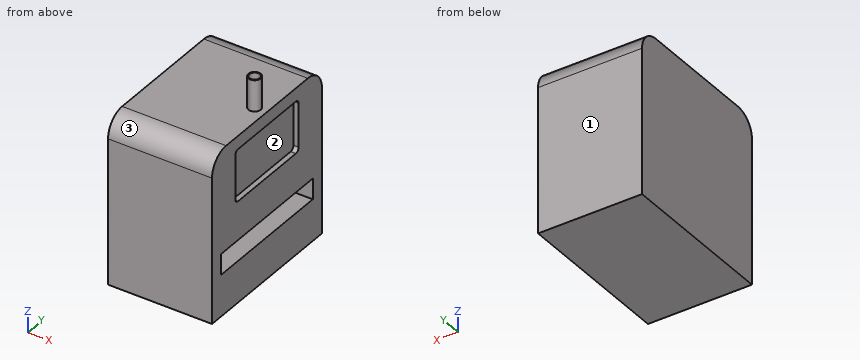
```python
from build123d import *

# Parameters (mm, degrees)
F0_W      = 780
F0_H      = 800
F1_DEPTH  = 500
F2_R      = 100
F3_R      = 30
F4_DEPTH  = 150
F5_R      = 25
F6_DEPTH  = 200
F7_W      = 450
F7_H      = 250
F8_DEPTH  = 25
F9_R      = 20
F11_DEPTH = 150


with BuildPart() as f1:
    # F0 (on Right) → F1 (new body)
    with BuildSketch(Plane.YZ):
        Rectangle(F0_W, F0_H)
    extrude(amount=-F1_DEPTH)

    # F2
    f2_edges = [f1.edges().sort_by_distance(p)[0] for p in [
        (-250, -390, 400),
        (-250, 390, 400),
    ]]
    fillet(f2_edges, radius=F2_R)

    # F3 (on face) → F4 (join)
    with BuildSketch(Plane.XY.offset(400)):
        with Locations((-59.408359, 0)):
            Circle(F3_R)
    extrude(amount=F4_DEPTH)

    # F5 (on face) → F6 (cut)
    with BuildSketch(Plane.XY.offset(550)):
        with Locations((-59.408359, 0)):
            Circle(F5_R)
    extrude(amount=-F6_DEPTH, mode=Mode.SUBTRACT)

    # F7 (on face) → F8 (cut)
    with BuildSketch(Plane.YZ):
        with Locations((0, 211.28722)):
            Rectangle(F7_W, F7_H)
    extrude(amount=-F8_DEPTH, mode=Mode.SUBTRACT)

    # F9
    f9_edges = [f1.edges().sort_by_distance(p)[0] for p in [
        (-12.5, -225, 336.28722),
        (-12.5, 225, 336.28722),
        (-12.5, -225, 86.28722),
        (-12.5, 225, 86.28722),
    ]]
    fillet(f9_edges, radius=F9_R)

    # F10 (on face) → F11 (cut)
    with BuildSketch(Plane.YZ):
        Polygon((0, -200), (325, -200), (325, -100), (-325, -100), (-325, -200), align=None)
    extrude(amount=-F11_DEPTH, mode=Mode.SUBTRACT)


solid = f1.part
```
Could you check a few things on this model? Use its own coordinates, in mm. Face numbers are marked on the shaded views. Coordinates: 2 decimals unless noted, no trailing zeros. Loops run counter-clockwise (first coordinate to the right, second up) from the corner with the lowest first, then second, coordinate; pieces in that order, holes last.
1) Imagine slicing it at D-D (z = 370). List the corners of the cut face in (x, y) for me, and give its area (3 significant figures).
Reported:
outline: (-500, -361.41) - (0, -361.41) - (0, 361.41) - (-500, 361.41) - close; hole circle Ø50 at (-59.41, 0)
area: 359,000 mm2
2) Imagine slicing it at A-A (y = 0). List the corners of the cut face in (x, z) for me.
Reported:
outline: (-500, -400) - (0, -400) - (0, -200) - (-150, -200) - (-150, -100) - (0, -100) - (0, 86.29) - (-25, 86.29) - (-25, 336.29) - (0, 336.29) - (0, 400) - (-29.41, 400) - (-29.41, 550) - (-34.41, 550) - (-34.41, 350) - (-84.41, 350) - (-84.41, 550) - (-89.41, 550) - (-89.41, 400) - (-500, 400) - close
3) Thinking about a two-plate mould opening in Z: for the marked faces 1, 2 and 3, which applies, released by +Z, released by -Z, zero draft, split by the parting line, or undercut?
Reported:
face 1: zero draft
face 2: undercut
face 3: released by +Z
4) Imagine slicing it at C-C (x = -349). List the corners of the cut face in (y, z) for me, and give its area (3 significant figures).
Reported:
outline: (-390, -400) - (390, -400) - (390, 300) arc R100 ccw to (290, 400) - (-290, 400) arc R100 ccw to (-390, 300) - close
area: 620,000 mm2
5) Will these pins go through, and if not, where does the flat tip stop? pin 1 Ø4 at (x, y) = (-369, 103.5) entering from +Z; pin 2 Ø15 at (x, y) = (-61.5, 5) entering from +Z.
Reported:
pin 1: stops at z = 400
pin 2: stops at z = 350
6) Please list where these lines run through material, in increasing order: line 1 along Z through (x, y) = (-146.5, 118); line 2 along Z through (x, y) = (-332, -82); line 3 along Z through (x, y) = (-190.5, -333.5).
Reported:
line 1: z = -400 to -200, -100 to 400
line 2: z = -400 to 400
line 3: z = -400 to 390.04
7) Imagine slicing it at B-B (x = -55). List the corners of the cut face in (y, z) for me.
Reported:
outline: (-390, -400) - (390, -400) - (390, 300) arc R100 ccw to (290, 400) - (29.67, 400) - (29.67, 550) - (24.61, 550) - (24.61, 350) - (-24.61, 350) - (-24.61, 550) - (-29.67, 550) - (-29.67, 400) - (-290, 400) arc R100 ccw to (-390, 300) - close; hole (-325, -200) - (325, -200) - (325, -100) - (-325, -100) - close
